The listing builds one solid part. Answer for the finished solid, in the listing's coordinates (mm). Face numbers are marked on the shaded views. A direction names the side the tool comes from. Give positions to 0.01 mm unless a question says otherwise; leave off trailing zeros. Order: outer loops, then holes, each group sorted by start corner. A loop starts at its lowest first (then second) coordinate and runs counter-clockwise, first axis right, second up. Notation, with made-up numbers: (10, -4) - (44, -4) arc R11 cw to (44, 14) - close; hole circle Ø6 at (26.5, -28.75). An arc over 180 degrees is marked (long way). Answer as CSV lines item,"result". Start each with the question number.
1. Section D-D on z = 0 is taken. Count the separate pieces of the cut face and the enclosed holes in it, and give its area (3 significant figures).
2. Section A-A on z = 27 is taken. Give the vertices of the cut face in (x, y), and give its area (3 significant figures).
3. Consider line 1 along Z through (x, y) = (54.85, 90); line 2 along Z through (x, y) = (54.2, 142); line 3 along X through (y, z) = (1.65, 17.5). Determine where each line is inside the solid, lowest interval first. Write a range as [from, to].
4. Section C-C on y = 42 is taken. Give the vertices of the cut face in (x, z), and give its area (3 significant figures).
5. Which of the six approach directions +Z, -Z, +X, -X, +Y, -Y give full straight-line access (tool end or side, diameter ignored) to the marked faces 1, 2 and 3?
6. Flat-ended cylindrical pins translate along their axes: pin 1 (1.2 mm diameter, centred on y = 12.5, z = 32.5, fed in from +X); pin 2 (8 mm diameter, centred on x = 14.5, z = 26, fed in from -Y); pin 3 (5.5 mm diameter, centred on y = 142, z = -9, fed in from +X); pin 4 (10 mm diameter, centred on x = -34, z = -4.5, fed in from +Y). Find the tip coordinate at first contact, or state that the pin passes through.
7. Section B-B on x = -67.75 is taken. Give the vertices of the cut face in (y, z), and give its area (3 significant figures).
8. Determine the mould class of the marked faces 4, 5 and 6 for opening direction X: +X half, -X half, draft (parallel to the pull), parting line (faces both ways), or undercut.
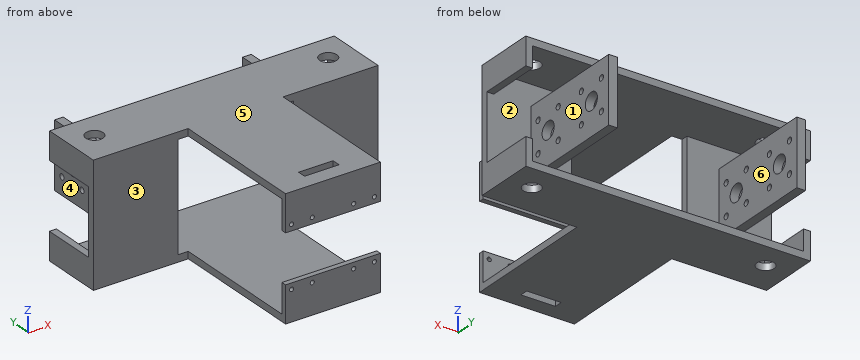
from build123d import *

# Parameters (mm, degrees)
SKETCH1_W                 = 75
SKETCH1_H                 = 40
SKETCH1_R                 = 5
SKETCH1_R_2               = 1.7
SKETCH1_W_2               = 10
SKETCH1_H_2               = 20
BOSS_EXTRUDE1_DEPTH       = 3
CUT_EXTRUDE1_DEPTH        = 43.605750786
CUT_EXTRUDE1_DEPTH_BACK   = 43.605750786
SKETCH2_W                 = 67
SKETCH2_H                 = 28
BOSS_EXTRUDE3_DEPTH       = 110
BOSS_EXTRUDE3_DEPTH_BACK  = 3
SKETCH6_W                 = 67
SKETCH6_H                 = 11
CUT_EXTRUDE4_DEPTH        = 122.372360939
SKETCH7_W                 = 70
SKETCH7_H                 = 37
BOSS_EXTRUDE4_DEPTH       = 45
SKETCH8_W                 = 45
SKETCH8_H                 = 62
CUT_EXTRUDE6_DEPTH        = 29
SKETCH11_W                = 45
SKETCH11_H                = 4
CUT_EXTRUDE9_DEPTH        = 157.445677473
SKETCH9_W                 = 38
SKETCH9_H                 = 28.5
CUT_EXTRUDE10_DEPTH       = 204.024629048
SKETCH13_W                = 5
SKETCH13_H                = 38
BOSS_EXTRUDE5_DEPTH       = 32
SKETCH14_R                = 5
SKETCH14_R_2              = 1.7
CUT_EXTRUDE11_DEPTH       = 32
SKETCH15_W                = 165
SKETCH15_H                = 70
SKETCH15_W_2              = 157
SKETCH15_H_2              = 62
BOSS_EXTRUDE6_DEPTH       = 3
SKETCH16_W                = 20
SKETCH16_H                = 4.820648258
CUT_EXTRUDE12_DEPTH       = 159.626132778
SKETCH18_R                = 5
CUT_EXTRUDE14_DEPTH       = 159.626132778
MIRROR6_COPY_1_SKETCH_W   = 5
MIRROR6_COPY_1_SKETCH_H   = 38
MIRROR6_COPY_1_DEPTH      = 32
MIRROR6_COPY_2_SKETCH_R   = 5
MIRROR6_COPY_2_SKETCH_R_2 = 1.7
MIRROR6_COPY_2_DEPTH      = 32
SKETCH19_W                = 38
SKETCH19_H                = 3.5
CUT_EXTRUDE15_DEPTH       = 10
SKETCH20_R                = 1.2
CUT_EXTRUDE16_DEPTH       = 10
SKETCH21_W                = 10
SKETCH21_H                = 80
CUT_EXTRUDE17_DEPTH       = 184.330984833


with BuildPart() as part:
    # Sketch1 → Boss-Extrude1 (new body)
    with BuildSketch(Plane(origin=(0, 0, 0), x_dir=(1, 0, 0), z_dir=(0, 1, 0))):
        Rectangle(SKETCH1_W, SKETCH1_H)
        with Locations(Location((-21, 0, 0), (0, 0, 270))):
            Circle(SKETCH1_R, mode=Mode.SUBTRACT)
        with Locations(Location((-30, 8.25, 0), (0, 0, 270))):
            Circle(SKETCH1_R_2, mode=Mode.SUBTRACT)
        with Locations(Location((-12, 8.25, 0), (0, 0, 270))):
            Circle(SKETCH1_R_2, mode=Mode.SUBTRACT)
        with Locations(Location((-12, -8.25, 0), (0, 0, 270))):
            Circle(SKETCH1_R_2, mode=Mode.SUBTRACT)
        with Locations(Location((-30, -8.25, 0), (0, 0, 270))):
            Circle(SKETCH1_R_2, mode=Mode.SUBTRACT)
        with Locations(Location((12, 8.25, 0), (0, 0, 90))):
            Circle(SKETCH1_R_2, mode=Mode.SUBTRACT)
        with Locations(Location((12, -8.25, 0), (0, 0, 90))):
            Circle(SKETCH1_R_2, mode=Mode.SUBTRACT)
        with Locations(Location((21, 0, 0), (0, 0, 90))):
            Circle(SKETCH1_R, mode=Mode.SUBTRACT)
        with Locations(Location((30, -8.25, 0), (0, 0, 90))):
            Circle(SKETCH1_R_2, mode=Mode.SUBTRACT)
        with Locations(Location((30, 8.25, 0), (0, 0, 90))):
            Circle(SKETCH1_R_2, mode=Mode.SUBTRACT)
        Rectangle(SKETCH1_W_2, SKETCH1_H_2, mode=Mode.SUBTRACT)
    extrude(amount=BOSS_EXTRUDE1_DEPTH)

    # Sketch2 → Cut-Extrude1 (cut, two sides: drawn at the far end of the back side and taken through both)
    with BuildSketch(Plane(origin=(0, 3, 0), x_dir=(1, 0, 0), z_dir=(0, 1, 0)).offset(-CUT_EXTRUDE1_DEPTH_BACK)):
        Rectangle(SKETCH2_W, SKETCH2_H)
    extrude(amount=CUT_EXTRUDE1_DEPTH + CUT_EXTRUDE1_DEPTH_BACK, mode=Mode.SUBTRACT)

    # Sketch3 → Boss-Extrude3 (add, two sides: drawn at the far end of the back side and taken through both)
    with BuildSketch(Plane(origin=(0, 3, 0), x_dir=(1, 0, 0), z_dir=(0, 1, 0)).offset(-BOSS_EXTRUDE3_DEPTH_BACK)):
        Polygon((37.5, -35), (37.5, -20), (33.5, -20), (-33.5, -20), (-37.5, -20), (-37.5, -35), align=None)
        Polygon((33.5, 20), (37.5, 20), (37.5, 35), (-37.5, 35), (-37.5, 20), (-33.5, 20), align=None)
        Polygon((37.5, -20), (37.5, 20), (33.5, 20), (33.5, 14), (33.5, -14), (33.5, -20), align=None)
        Polygon((-33.5, 14), (-33.5, 20), (-37.5, 20), (-37.5, -20), (-33.5, -20), (-33.5, -14), align=None)
    extrude(amount=BOSS_EXTRUDE3_DEPTH + BOSS_EXTRUDE3_DEPTH_BACK)

    # Sketch6 → Cut-Extrude4 (cut, through all)
    with BuildSketch(Plane(origin=(0, 3, 0), x_dir=(1, 0, 0), z_dir=(0, 1, 0))):
        with Locations((0, -25.5)):
            Rectangle(SKETCH6_W, SKETCH6_H)
        with Locations((0, 25.5)):
            Rectangle(SKETCH6_W, SKETCH6_H)
    extrude(amount=CUT_EXTRUDE4_DEPTH, mode=Mode.SUBTRACT)

    # Sketch7 → Boss-Extrude4 (add)
    with BuildSketch(Plane.ZY.offset(37.5)):
        with Locations((0, 94.5)):
            Rectangle(SKETCH7_W, SKETCH7_H)
    boss_extrude4 = extrude(amount=BOSS_EXTRUDE4_DEPTH)

    # Mirror2: Boss-Extrude4 across plane
    add(boss_extrude4.mirror(Plane(origin=(0, 0, 0), x_dir=(0, 0, 1), z_dir=(1, 0, 0))))

    # Sketch8 → Cut-Extrude6 (cut)
    with BuildSketch(Plane(origin=(0, 113, 0), x_dir=(1, 0, 0), z_dir=(0, 1, 0))):
        with Locations((-56, 0)):
            Rectangle(SKETCH8_W, SKETCH8_H)
        with Locations((56, 0)):
            Rectangle(SKETCH8_W, SKETCH8_H)
    extrude(amount=-CUT_EXTRUDE6_DEPTH, mode=Mode.SUBTRACT)

    # Sketch11 → Cut-Extrude9 (cut, through all)
    with BuildSketch(Plane.XY.offset(35)):
        with Locations((-60, 78)):
            Rectangle(SKETCH11_W, SKETCH11_H)
        with Locations((60, 78)):
            Rectangle(SKETCH11_W, SKETCH11_H)
    extrude(amount=-CUT_EXTRUDE9_DEPTH, mode=Mode.SUBTRACT)

    # Sketch9 → Cut-Extrude10 (cut, through all)
    with BuildSketch(Plane.ZY.offset(82.5)):
        with Locations((0, 98.25)):
            Rectangle(SKETCH9_W, SKETCH9_H)
    extrude(amount=-CUT_EXTRUDE10_DEPTH, mode=Mode.SUBTRACT)

    # Sketch13 → Boss-Extrude5 (add)
    with BuildSketch(Plane(origin=(0, 84, 0), x_dir=(1, 0, 0), z_dir=(0, 1, 0))):
        with Locations((-54.5, 0)):
            Rectangle(SKETCH13_W, SKETCH13_H)
    boss_extrude5 = extrude(amount=BOSS_EXTRUDE5_DEPTH)

    # Sketch14 → Cut-Extrude11 (cut)
    with BuildSketch(Plane.ZY.offset(57)):
        with Locations((0, 98.25)):
            Circle(SKETCH14_R)
        with Locations((-9, 106.5)):
            Circle(SKETCH14_R_2)
        with Locations((9, 106.5)):
            Circle(SKETCH14_R_2)
        with Locations((9, 90)):
            Circle(SKETCH14_R_2)
        with Locations((-9, 90)):
            Circle(SKETCH14_R_2)
    cut_extrude11 = extrude(amount=-CUT_EXTRUDE11_DEPTH, mode=Mode.SUBTRACT)

    # Mirror4: Boss-Extrude5, Cut-Extrude11 across plane
    add(boss_extrude5.mirror(Plane(origin=(0, 0, 0), x_dir=(0, 0, 1), z_dir=(1, 0, 0))))
    add(cut_extrude11.mirror(Plane(origin=(0, 0, 0), x_dir=(0, 0, 1), z_dir=(1, 0, 0))), mode=Mode.SUBTRACT)

    # Sketch15 → Boss-Extrude6 (add)
    with BuildSketch(Plane(origin=(0, 113, 0), x_dir=(1, 0, 0), z_dir=(0, 1, 0))):
        Rectangle(SKETCH15_W, SKETCH15_H)
        Rectangle(SKETCH15_W_2, SKETCH15_H_2, mode=Mode.SUBTRACT)
    extrude(amount=BOSS_EXTRUDE6_DEPTH)

    # Sketch16 → Cut-Extrude12 (cut, through all)
    with BuildSketch(Plane.XY.offset(35)):
        with Locations((0, 11.636111214)):
            Rectangle(SKETCH16_W, SKETCH16_H)
    extrude(amount=-CUT_EXTRUDE12_DEPTH, mode=Mode.SUBTRACT)

    # Sketch18 → Cut-Extrude14 (cut, through all)
    with BuildSketch(Plane.XY.offset(35)):
        with Locations((67.75, 100)):
            Circle(SKETCH18_R)
    cut_extrude14 = extrude(amount=-CUT_EXTRUDE14_DEPTH, mode=Mode.SUBTRACT)

    # Mirror5: Cut-Extrude14 across plane
    add(cut_extrude14.mirror(Plane(origin=(0, 0, 0), x_dir=(0, 0, 1), z_dir=(1, 0, 0))), mode=Mode.SUBTRACT)

    # Mirror6: Boss-Extrude5, Cut-Extrude11 across plane
    add(boss_extrude5.mirror(Plane.ZX.offset(116)))
    add(cut_extrude11.mirror(Plane.ZX.offset(116)), mode=Mode.SUBTRACT)

    # Mirror6 copy 1 sketch → Mirror6 copy 1 (add)
    with BuildSketch(Plane(origin=(0, 148, 0), x_dir=(-1, 0, 0), z_dir=(0, -1, 0))):
        with Locations((-54.5, 0)):
            Rectangle(MIRROR6_COPY_1_SKETCH_W, MIRROR6_COPY_1_SKETCH_H)
    extrude(amount=MIRROR6_COPY_1_DEPTH)

    # Mirror6 copy 2 sketch → Mirror6 copy 2 (cut)
    with BuildSketch(Plane(origin=(57, 232, 0), x_dir=(0, 0, 1), z_dir=(1, 0, 0))):
        with Locations((0, 98.25)):
            Circle(MIRROR6_COPY_2_SKETCH_R)
        with Locations((-9, 106.5)):
            Circle(MIRROR6_COPY_2_SKETCH_R_2)
        with Locations((9, 106.5)):
            Circle(MIRROR6_COPY_2_SKETCH_R_2)
        with Locations((9, 90)):
            Circle(MIRROR6_COPY_2_SKETCH_R_2)
        with Locations((-9, 90)):
            Circle(MIRROR6_COPY_2_SKETCH_R_2)
    extrude(amount=-MIRROR6_COPY_2_DEPTH, mode=Mode.SUBTRACT)

    # Sketch19 → Cut-Extrude15 (cut)
    with BuildSketch(Plane(origin=(82.5, 0, 0), x_dir=(0, 0, -1), z_dir=(1, 0, 0))):
        with Locations((0, 114.25)):
            Rectangle(SKETCH19_W, SKETCH19_H)
    cut_extrude15 = extrude(amount=-CUT_EXTRUDE15_DEPTH, mode=Mode.SUBTRACT)

    # Mirror7: Cut-Extrude15 across plane
    add(cut_extrude15.mirror(Plane(origin=(0, 0, 0), x_dir=(0, 0, 1), z_dir=(1, 0, 0))), mode=Mode.SUBTRACT)

    # Sketch20 → Cut-Extrude16 (cut)
    with BuildSketch(Plane(origin=(0, 3, 0), x_dir=(1, 0, 0), z_dir=(0, 1, 0))):
        with Locations(Location((-24, 17.5, 0), (0, 0, 270))):
            Circle(SKETCH20_R)
        with Locations(Location((-12, 17.5, 0), (0, 0, 270))):
            Circle(SKETCH20_R)
        with Locations(Location((12, 17.5, 0), (0, 0, 270))):
            Circle(SKETCH20_R)
        with Locations(Location((-24, -17.5, 0), (0, 0, 270))):
            Circle(SKETCH20_R)
        with Locations(Location((-12, -17.5, 0), (0, 0, 270))):
            Circle(SKETCH20_R)
        with Locations(Location((24, 17.5, 0), (0, 0, 270))):
            Circle(SKETCH20_R)
        with Locations(Location((12, -17.5, 0), (0, 0, 270))):
            Circle(SKETCH20_R)
        with Locations(Location((24, -17.5, 0), (0, 0, 270))):
            Circle(SKETCH20_R)
    extrude(amount=-CUT_EXTRUDE16_DEPTH, mode=Mode.SUBTRACT)

    # Sketch21 → Cut-Extrude17 (cut, through all)
    with BuildSketch(Plane.XY.offset(35)):
        with Locations((32.5, 40)):
            Rectangle(SKETCH21_W, SKETCH21_H)
        with Locations((-32.5, 40)):
            Rectangle(SKETCH21_W, SKETCH21_H)
    extrude(amount=-CUT_EXTRUDE17_DEPTH, mode=Mode.SUBTRACT)


solid = part.part
Checks:
1,separate pieces,"6"
1,enclosed holes,"0"
1,area,"832 mm²"
2,outline,"(-82.5, 80) - (-33.5, 80) - (-33.5, 84) - (-78.5, 84) - (-78.5, 116) - (-82.5, 116) - close; (-27.5, 0) - (27.5, 0) - (27.5, 3) - (-27.5, 3) - close; (33.5, 80) - (82.5, 80) - (82.5, 116) - (78.5, 116) - (78.5, 84) - (33.5, 84) - close"
2,area,"813 mm²"
3,line 1,"z = [-35, -31], [-19, -10.7], [-7.3, 7.3], [10.7, 19], [31, 35]"
3,line 2,"z = [-19, -10.7], [-7.3, 7.3], [10.7, 19]"
3,line 3,"x = [-27.5, -25.2], [-22.8, -13.2], [-10.8, 10.8], [13.2, 22.8], [25.2, 27.5]"
4,outline,"(-27.5, -35) - (27.5, -35) - (27.5, -31) - (-27.5, -31) - close; (-27.5, 31) - (27.5, 31) - (27.5, 35) - (-27.5, 35) - close"
4,area,"440 mm²"
5,face 1,"+X, +Y"
5,face 2,"+Y"
5,face 3,"+Z, -Z, -X, -Y"
6,pin 1,"stops at x = 27.5"
6,pin 2,"stops at y = 0"
6,pin 3,"stops at x = 57"
6,pin 4,"stops at y = 84"
7,outline,"(80, -35) - (95, -35) - (95, -31) - (84, -31) - (84, 31) - (95, 31) - (95, 35) - (80, 35) - close; (105, -35) - (116, -35) - (116, -31) - (105, -31) - close; (105, 31) - (116, 31) - (116, 35) - (105, 35) - close"
7,area,"456 mm²"
8,face 4,"-X half"
8,face 5,"draft"
8,face 6,"undercut"
